For this review, use the dimensioned drawing (mm, ordinates from the lowest corner) and the shaded views. A direction names the side the tool comes from. Give positions to 0.01 mm unless a question says otherwise; leave off trailing zeros. Order: outer loops, then holes, each group sorted by start corner. A loop starts at its lowest first (then second) coordinate and runs counter-clockwise, first axis right, second up. Notation, with made-up numbers: (-39.75, 63) - (-18.75, 63) arc R21 ccw to (-18.75, 78) - close; hole circle Ø7 at (-17, 53.5). An arc over 180 degrees is marked (long way). One line per item, written item: value.
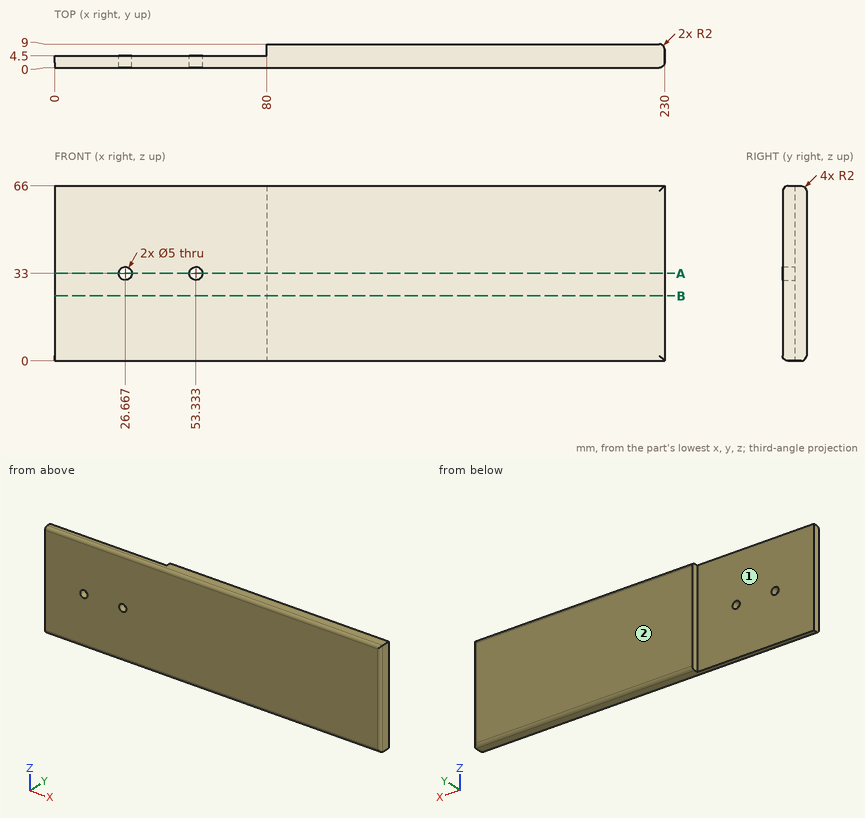
(1) Wall thickness on line 1 (X direction, y = 2.75, z = 33); line 2 (X direction, y = 1.1, z = 33) (1 decimal); line 3 (Z direction, x = 31, y = 1.75) (1 decimal): over which ranges is each line inside the solid? List them lowest first. Write a range as from..to.
Answers below:
line 1: x = 0..24.17, 29.17..50.83, 55.83..230
line 2: x = 0..24.2, 29.2..50.8, 55.8..229.8
line 3: z = 0..66
(2) Machinability: for the marked faces 1 and 2, which of the approach directions +Z, -Z, +X, -X, +Y, -Y give a long, thin tool a straight path to every point of the face, cutting with its end or side? Answer none if there is none.
Answers below:
face 1: +Z, -Z, -X, +Y
face 2: +Z, -Z, +X, -X, +Y
(3) Take a section at B-B (z = 24.5). Write out the cut boundary in (x, y), then the cut area to 3 significant figures.
Answers below:
outline: (0, 0) - (228, 0) arc R2 ccw to (230, 2) - (230, 7) arc R2 ccw to (228, 9) - (80, 9) - (80, 4.5) - (0, 4.5) - close
area: 1,710 mm^2
(4) Take a section at A-A (z = 33). Write out the cut boundary in (x, y).
Answers below:
outline: (0, 0) - (24.17, 0) - (24.17, 4.5) - (0, 4.5) - close; (29.17, 0) - (50.83, 0) - (50.83, 4.5) - (29.17, 4.5) - close; (55.83, 0) - (228, 0) arc R2 ccw to (230, 2) - (230, 7) arc R2 ccw to (228, 9) - (80, 9) - (80, 4.5) - (55.83, 4.5) - close
(5) For P1, Ø3.5, axis at y = 7, z = 40.5, coming from the -X side; P2, Ø8, axis at x = 26.67, z = 33, coming from the +Y side; P3, Ø1.5, axis at x = 168, y = 8, coming from the -Z side; P4, Ø4.5, axis at x = 53.33, z = 33, coming from the +Y side, all flat-tipped, find the tip position at first contact; note any pin that passes through.
Answers below:
P1: stops at x = 80
P2: stops at y = 4.5
P3: stops at z = 0.02
P4: passes through
